Source: CAD feature listing. Evaluate the final solid. Frame: model axes, mm. A direction names the side the tool comes from. Coordinates: 2 decimals unless noted, no trailing zeros. Order: outer loops, then holes, each group sorted by start corner. A loop starts at its lowest first (then second) coordinate and runs counter-clockwise, first axis right, second up.
```python
from build123d import *

# Parameters (mm, degrees)
F_6_0MM_DOWEL_HOLE7_D     = 6
F_6_0MM_DOWEL_HOLE7_DEPTH = 12
F_6_0MM_DOWEL_HOLE7_TIP   = 3
CUT_EXTRUDE1_DEPTH        = 9.2
CUT_EXTRUDE1_DEPTH_BACK   = 9.2
FILLET1_R                 = 2
FILLET2_R                 = 2
FILLET6_R                 = 1
FILLET7_R                 = 1
BOSS_EXTRUDE1_DEPTH       = 10
BOSS_EXTRUDE1_DEPTH_BACK  = 10
FILLET8_R                 = 1


with BuildPart() as part:
    # Sketch1 → Revolve1 (revolve)
    with BuildSketch(Plane.XY, mode=Mode.PRIVATE) as revolve1_sk:
        Polygon((0, 0), (40, 0), (40, -16), (15, -42), (0, -42), align=None)
    revolve(revolve1_sk.sketch.rotate(Axis((0, -42, 0), (0, 1, 0)), 90), axis=Axis((0, -42, 0), (0, 1, 0)))

    # 6.0mm Dowel Hole7
    with Locations(Plane(origin=(0, 0, 0), x_dir=(1, 0, 0), z_dir=(0, 1, 0))):
        with Locations((20, -20), (-20, 20), (-20, -20), (20, 20)):
            Hole(F_6_0MM_DOWEL_HOLE7_D / 2, depth=F_6_0MM_DOWEL_HOLE7_DEPTH)
            with Locations((0, 0, -(F_6_0MM_DOWEL_HOLE7_DEPTH + F_6_0MM_DOWEL_HOLE7_TIP / 2))):  # 90° drill point
                Cone(0, F_6_0MM_DOWEL_HOLE7_D / 2, F_6_0MM_DOWEL_HOLE7_TIP, mode=Mode.SUBTRACT)

    # Sketch13 → Cut-Extrude1 (cut, two sides: drawn at the far end of the back side and taken through both)
    with BuildSketch(Plane.XY.offset(-CUT_EXTRUDE1_DEPTH_BACK)):
        Polygon((-2.55, 0), (2.55, 0), (2.55, -20), (1, -40), (-1, -40), (-2.55, -20), align=None)
    extrude(amount=CUT_EXTRUDE1_DEPTH + CUT_EXTRUDE1_DEPTH_BACK, mode=Mode.SUBTRACT)

    # Fillet1
    fillet1_edges = [part.edges().sort_by_distance(p)[0] for p in [
        (0, -42, 15),
    ]]
    fillet(fillet1_edges, radius=FILLET1_R)

    # Fillet2
    fillet2_edges = [part.edges().sort_by_distance(p)[0] for p in [
        (0, -16, 40),
    ]]
    fillet(fillet2_edges, radius=FILLET2_R)

    # Fillet6
    fillet6_edges = [part.edges().sort_by_distance(p)[0] for p in [
        (1, -40, 0),
    ]]
    fillet(fillet6_edges, radius=FILLET6_R)

    # Fillet7
    fillet7_edges = [part.edges().sort_by_distance(p)[0] for p in [
        (-1, -40, 0),
    ]]
    fillet(fillet7_edges, radius=FILLET7_R)

    # Sketch14 → Boss-Extrude1 (add, two sides: drawn at the far end of the back side and taken through both)
    with BuildSketch(Plane(origin=(0, 0, 0), x_dir=(0, 0, -1), z_dir=(1, 0, 0)).offset(-BOSS_EXTRUDE1_DEPTH_BACK)):
        Polygon((9.2, -30), (12.2, -27), (9.2, -24), (6.2, -27), align=None)
    extrude(amount=BOSS_EXTRUDE1_DEPTH + BOSS_EXTRUDE1_DEPTH_BACK)

    # Fillet8
    fillet8_edges = [part.edges().sort_by_distance(p)[0] for p in [
        (0, -27, -6.2),
    ]]
    fillet(fillet8_edges, radius=FILLET8_R)


solid = part.part
```
1. Section query B-B on y = -32. Return loops of the section in (x, z), plus the area to 3 significant figures.
Findings:
outline: circle Ø49.23 at (0, 0); hole (-1.62, -9.2) - (1.62, -9.2) - (1.62, 9.2) - (-1.62, 9.2) - close
area: 1,840 mm2
2. Ray query, line 1 (Z direction, x = 20, y = -5); line 2 (X direction, y = -2.5, z = 18). Return the intervals inside material, ascending.
Findings:
line 1: z = -34.64 to -23, -17 to 17, 23 to 34.64
line 2: x = -35.72 to -22.24, -17.76 to 17.76, 22.24 to 35.72
3. Access query for faces 4 (the face through (2.55, -10, 0)), 5 (the face through (0, -35, -9.2)), 6 (the face through (-12.015, -7.704, -38.153)). Directions: +Z, -Z, +X, -X, +Y, -Y. A direction counts if a zero-diameter tool reaches every point of the face in a straight line with its end or side. Return the directions, or none.
Findings:
face 4: +Y
face 5: none
face 6: +Y, -Y
4. Section query A-A on y = -7. Return loops of the section in (x, z), plus the area to 3 significant figures.
Findings:
outline: circle Ø80 at (0, 0); hole circle Ø6 at (-20, -20); hole circle Ø6 at (-20, 20); hole (-2.55, -9.2) - (2.55, -9.2) - (2.55, 9.2) - (-2.55, 9.2) - close; hole circle Ø6 at (20, -20); hole circle Ø6 at (20, 20)
area: 4,820 mm2
5. Pin query (flat end, axial travel): P1, Ø12, axis at y = -9.5, z = -7.5, coming from the +X side; P2, Ø5, axis at x = -20, z = -20, coming from the +Y side; P3, Ø6, axis at x = 17.5, y = -36.5, coming from the +Z side. Return the tip coordinate at first contact, or that it passes through.
Findings:
P1: stops at x = 39.97
P2: stops at y = -12.5
P3: stops at z = 16.25
6. Draft query along Y for faces 1 (the face through (-17.6, -6.1, -18.2)), 2 (the face through (0, -25.1, -8.1)), 3 (the face through (0, -28.8, -8)). Return one class per face: released by +Y, released by -Y, zero draft, split by the parting line, or undercut.
Findings:
face 1: zero draft
face 2: released by +Y
face 3: undercut
